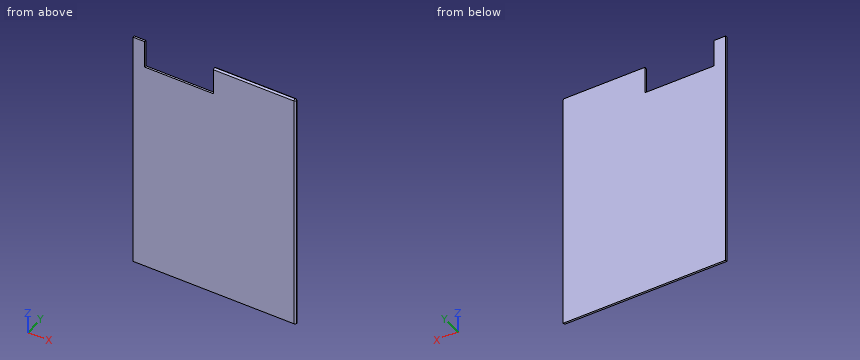
```python
from build123d import *

# Parameters (mm, degrees)
F1_DEPTH = 12.7
F2_R     = 10.16
F3_R     = 10.16


with BuildPart() as f1:
    # F0 (on Front) → F1 (new body)
    with BuildSketch(Plane.XZ):
        Polygon((-538.48, -812.8), (538.48, -812.8), (538.48, 812.8), (-5.08, 812.8), (-5.08, 628.65), (-462.28, 628.65), (-462.28, 812.8), (-538.48, 812.8), align=None)
    extrude(amount=F1_DEPTH)

    # F2
    f2_edges = [f1.edges().sort_by_distance(p)[0] for p in [
        (266.7, -12.7, 812.8),
    ]]
    fillet(f2_edges, radius=F2_R)

    # F3
    f3_edges = [f1.edges().sort_by_distance(p)[0] for p in [
        (538.48, -12.7, -5.08),
    ]]
    fillet(f3_edges, radius=F3_R)


solid = f1.part
```
Source: CAD feature listing. Evaluate the final solid. Frame: model axes, mm. Coordinates: 2 decimals unless noted, no trailing zeros. Loops run counter-clockwise (first coordinate to the right, second up) from the corner with the lowest first, then second, coordinate; pieces in that order, holes last. Notation, with made-up numbers: M 52,41 L 85,41 A20 ccw 85,45 Z; hole C 19,50.5 d3. An arc over 180 degrees is marked long. Put each result on its own line as item: value. Start each with the question number.
1) Cut plane B-B on y = -6.5. Return the cut outline in (x, z), then the cut area to 3 significant figures.
2) Contact query for a flat-ended pin moving along its axis: pin 1 Ø4 at (y, z) = (-7, 746) entering from +X. Output: stop coordinate, or through.
3) Ray query, L1, parallel to X at y = -3.75, z = 693; L2, parallel to Z at x = -383.5, y = -5.5; L3, parallel to X at y = -3.75, z = 448. Return the intervals inside material, ascending. Write a range as from..to.
4) Cut plane A-A on x = -439. Return the cut outline in (y, z).
The answers:
1. outline: M -538.48,-812.8 L 537.68,-812.8 L 537.68,802.64 A9.36 ccw 528.32,812 L -5.08,812 L -5.08,628.65 L -462.28,628.65 L -462.28,812.8 L -538.48,812.8 Z
1. area: 1,660,000 mm²
2. pin 1: stops at x = 538.18
3. L1: x = -538.48..-462.28, -5.08..538.41
3. L2: z = -812.8..628.65
3. L3: x = -538.48..538.41
4. outline: M -12.7,-812.8 L 0,-812.8 L 0,628.65 L -12.7,628.65 Z
